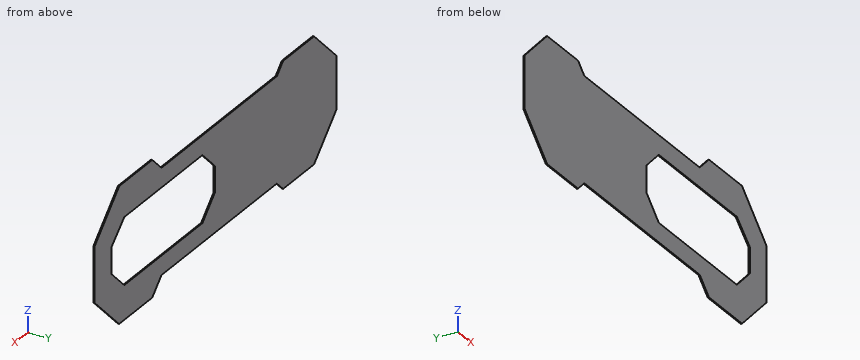
```python
from build123d import *

# Parameters (mm, degrees)
SM_BASE_FLANGE_1_DEPTH = 1
CUT_EXTRUDE_1_DEPTH    = 10


# Sheet-metal steps are written as plain solids
with BuildPart() as part:
    # Sketch 1 → Базовая кромка1 (new body)
    with BuildSketch(Plane(origin=(0, 0, 0), x_dir=(1, 0, 0), z_dir=(0, 1, 0))):
        Polygon((-57.720952925, -161.889640506), (-213.157461064, -161.889640506), (-213.778781408, -161.889640506), (-214.218121236, -161.450300678), (-222.278781408, -153.389640506), (-264.356991895, -153.389640506), (-295.11077987, -184.143428482), (-295.11077987, -227.635852531), (-264.356991895, -258.389640506), (-222.278781408, -258.389640506), (-214.218121236, -250.328980334), (-213.778781408, -249.889640506), (-213.157461064, -249.889640506), (-57.720952925, -249.889640506), (-57.099632582, -249.889640506), (-56.660292754, -250.328980334), (-44.599632582, -262.389640506), (0.278072842, -262.389640506), (33.88922013, -228.778493218), (33.88922013, -182.800787794), (0.478072842, -149.389640506), (-44.599632582, -149.389640506), (-56.660292754, -161.450300678), (-57.099632582, -161.889640506), align=None)
    extrude(amount=-SM_BASE_FLANGE_1_DEPTH)

    # Эскиз3 → Вырез-Вытянуть1 (cut)
    with BuildSketch(Plane(origin=(0, 0, 0), x_dir=(1, 0, 0), z_dir=(0, 1, 0))):
        Polygon((-129.650630124, -194.854768426), (-112.66234875, -177.866487052), (-6.632911498, -177.866487052), (10.895241956, -195.394640506), (10.895241956, -217.265248922), (-6.633389706, -233.712753004), (-112.662389706, -233.712753004), (-129.650630124, -216.724512586), align=None)
    extrude(amount=-CUT_EXTRUDE_1_DEPTH, mode=Mode.SUBTRACT)


solid = part.part
```
Could you check a few things on this model? Use its own coordinates, in mm. Round coordinates to 2 decimals unless told otherwise and drop trailing zeros. Order: outer loops, then holes, each group sorted by start corner. A loop starts at its lowest first (then second) coordinate and runs counter-clockwise, first axis right, second up. Notation, with made-up numbers: M 10.25,8.25 L 35.25,8.25 A15 ccw 35.25,16.25 Z; hole C 17.5,28.25 d5. An arc over 180 degrees is marked long. One line per question, with ' | ' between items. Start each with the question number.
(1) Suppose I cut it at A-A on z = 205. List the corners of the cut face in (x, y) for me.
(2) Please list where these lines run through material, in increasing order: line 1 along X through (y, z) = (-0.85, 203); line 2 along Z through (x, y) = (-35, -0.05); line 3 along Z through (x, y) = (-101, -0.85).
(3) Suppose I cut it at D-D on z = 171. List the corners of the cut face in (x, y) for me, then the cut area to 3 significant figures.
(4) For P1, Ø0.5, axis at x = -59.5, y = -0.5, coming from the -Z side; P2, Ø0.5, axis at x = -235, y = -0.5, coming from the -Z side; P3, Ø0.5, axis at x = -141, y = -0.5, coming from the +Z side, each with a flat end and sliding along its axis, tell me the tip position at first contact or that it passes through.
(5) Suppose I cut it at C-C on x = -175.5. List the corners of the cut face in (y, z) for me.
(6) Suppose I cut it at B-B on y = -0.5. List the corners of the cut face in (x, z) for me, then the cut area to 3 significant figures.
Geometry results:
1) outline: M -295.11,-1 L -129.65,-1 L -129.65,0 L -295.11,0 Z; M 10.9,-1 L 33.89,-1 L 33.89,0 L 10.9,0 Z
2) line 1: -295.11 to -129.65, 10.9 to 33.89 | line 2: 149.39 to 177.87, 233.71 to 262.39 | line 3: 161.89 to 177.87, 233.71 to 249.89
3) outline: M -281.97,-1 L 22.09,-1 L 22.09,0 L -281.97,0 Z | area: 304 mm²
4) P1: z = 161.89 | P2: z = 153.39 | P3: z = 249.89
5) outline: M -1,161.89 L 0,161.89 L 0,249.89 L -1,249.89 Z
6) outline: M -295.11,184.14 L -264.36,153.39 L -222.28,153.39 L -213.78,161.89 L -57.1,161.89 L -44.6,149.39 L 0.48,149.39 L 33.89,182.8 L 33.89,228.78 L 0.28,262.39 L -44.6,262.39 L -57.1,249.89 L -213.78,249.89 L -222.28,258.39 L -264.36,258.39 L -295.11,227.64 Z; hole M -129.65,194.85 L -112.66,177.87 L -6.63,177.87 L 10.9,195.39 L 10.9,217.27 L -6.63,233.71 L -112.66,233.71 L -129.65,216.72 Z | area: 23,000 mm²
